```python
from build123d import *

# Parameters (mm, degrees)
ESBO_O1_R             = 11
EXTRUS_O1_DEPTH       = 50
ESBO_O2_R             = 13
CORTE_EXTRUS_O1_DEPTH = 40
ESBO_O3_R             = 14.5
EXTRUS_O2_DEPTH       = 3


with BuildPart() as part:
    # Esboço1 → Extrusão1 (new body)
    with BuildSketch(Plane(origin=(0, 0, 0), x_dir=(0, 0, -1), z_dir=(1, 0, 0))):
        Circle(ESBO_O1_R)
    extrude(amount=-EXTRUS_O1_DEPTH)

    # Esboço2 → Corte-extrusão1 (cut, symmetric)
    with BuildSketch(Plane.XY):
        with Locations((-46, 0)):
            Circle(ESBO_O2_R)
    extrude(amount=CORTE_EXTRUS_O1_DEPTH, both=True, mode=Mode.SUBTRACT)

    # Esboço3 → Extrusão2 (add)
    with BuildSketch(Plane(origin=(0, 0, 0), x_dir=(0, 0, -1), z_dir=(1, 0, 0))):
        Circle(ESBO_O3_R)
    extrude(amount=EXTRUS_O2_DEPTH)


solid = part.part
```
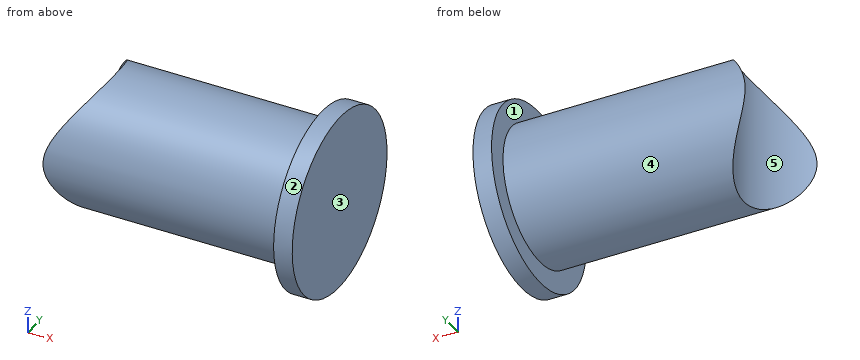
For this review, take the finished solid that the model builds, in its own axes (mm). Face numbers are marked on the shaded views. A direction names the side the tool comes from. Coordinates: 2 decimals unless noted, no trailing zeros. Loops run counter-clockwise (first coordinate to the right, second up) from the corner with the lowest first, then second, coordinate; pieces in that order, holes last. Notation, with made-up numbers: (27.25, 27.5) -> (76.25, 27.5) arc R14 ccw to (76.25, 54.5) -> close; hole circle Ø6 at (29, 81.5). An arc over 180 degrees is marked (long way). Return JSON: item names as keys, results as strings. Group by question number.
(1) Consider section D-D, the plane y = -12.5. Give the boundary of the cut face in (x, z).
(2) Consider section B-B, the plane y = 0. Give the boundary of the cut face in (x, z), plus the area to 3 significant figures.
(3) Consider section C-C, the plane x = -21.5. Give the boundary of the cut face in (y, z).
(4) Tool access review of the marked faces 1 and 2: name each direction out of +Z, -Z, +X, -X, +Y, -Y from which nothing blocks a thin tool from reaching the whole face with its end or side.
(5) For pin 1 Ø8.5 at (y, z) = (-3, -5.5) entering from -X; pin 2 Ø6 at (y, z) = (2.5, 7.5) entering from -X; pin 3 Ø1.5 at (y, z) = (2, 2) entering from -X; pin 4 Ø8 at (y, z) = (-8, 1) entering from -X, all flat-tipped, find the tip position at first contact; note any pin that passes through.
(6) Consider section A-A, the plane z = 0. Give the boundary of the cut face in (x, y).
(7) Mouldability with a two-part tool opening along Y and no side actions: class the marked faces 3, 4 and 5 as pulls with the +Y half, pulls with the -Y half, needs draft (parallel to the pull), parting line crosses it, or undercut.
(8) To check wall thickness, follow L1, parallel to Z at x = -24, y = 0.25; L2, parallel to X at y = 4, z = 13.75; L3, parallel to Y at x = -9, z = 0.5. State the ranges of each line that lie inside material, in increasing order.
Results below:
{
 "1": {"outline": "(0, -7.35) -> (3, -7.35) -> (3, 7.35) -> (0, 7.35) -> close"},
 "2": {"outline": "(-33, -11) -> (0, -11) -> (0, -14.5) -> (3, -14.5) -> (3, 14.5) -> (0, 14.5) -> (0, 11) -> (-33, 11) -> close", "area": "813 mm2"},
 "3": {"outline": "circle Ø22 at (0, 0)"},
 "4": {"face 1": "-X", "face 2": "+X, -X"},
 "5": {"pin 1": "stops at x = -35.21", "pin 2": "stops at x = -34.22", "pin 3": "stops at x = -33.29", "pin 4": "stops at x = -39.07"},
 "6": {"outline": "(-39.07, -11) -> (0, -11) -> (0, -14.5) -> (3, -14.5) -> (3, 14.5) -> (0, 14.5) -> (0, 11) -> (-39.07, 11) arc R13 cw to start"},
 "7": {"face 3": "needs draft", "face 4": "parting line crosses it", "face 5": "undercut"},
 "8": {"L1": "z = -11 to 11", "L2": "x = 0 to 3", "L3": "y = -10.99 to 10.99"}
}
